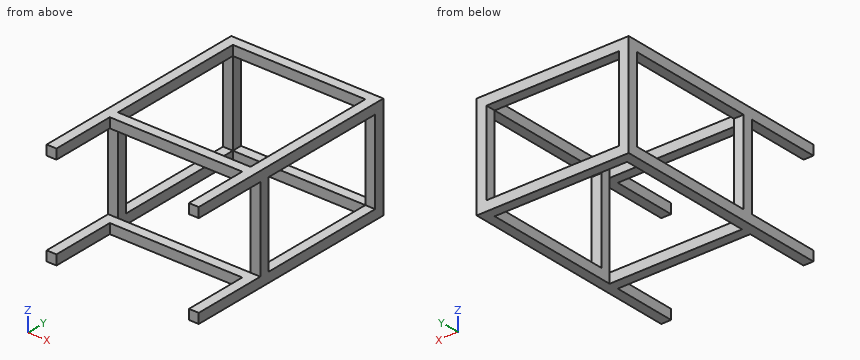
```python
from build123d import *

# Parameters (mm, degrees)
SKETCH_1_W          = 310
SKETCH_1_H          = 210
SKETCH_1_W_2        = 270
SKETCH_1_H_2        = 170
EXTRUDE_1_DEPTH     = 450
SKETCH_8_W          = 170
SKETCH_8_H          = 260
CUT_EXTRUDE_3_DEPTH = 310
SKETCH_11_W         = 170
SKETCH_11_H         = 150
CUT_EXTRUDE_4_DEPTH = 310
SKETCH_13_W         = 270
SKETCH_13_H         = 130
CUT_EXTRUDE_5_DEPTH = 521.216301167
SKETCH_14_W         = 270
SKETCH_14_H         = 280
CUT_EXTRUDE_6_DEPTH = 525.332909515


with BuildPart() as part:
    # 草图1 → 凸台-拉伸1 (new body)
    with BuildSketch(Plane(origin=(0, 0, 0), x_dir=(1, 0, 0), z_dir=(0, 1, 0))):
        Rectangle(SKETCH_1_W, SKETCH_1_H)
        Rectangle(SKETCH_1_W_2, SKETCH_1_H_2, mode=Mode.SUBTRACT)
    extrude(amount=EXTRUDE_1_DEPTH)

    # 草图8 → 切除-拉伸3 (cut)
    with BuildSketch(Plane(origin=(155, 0, 0), x_dir=(0, 0, -1), z_dir=(1, 0, 0))):
        with Locations((0, 300)):
            Rectangle(SKETCH_8_W, SKETCH_8_H)
    extrude(amount=-CUT_EXTRUDE_3_DEPTH, mode=Mode.SUBTRACT)

    # 草图11 → 切除-拉伸4 (cut)
    with BuildSketch(Plane(origin=(155, 0, 0), x_dir=(0, 0, -1), z_dir=(1, 0, 0))):
        with Locations((0, 75)):
            Rectangle(SKETCH_11_W, SKETCH_11_H)
    extrude(amount=-CUT_EXTRUDE_4_DEPTH, mode=Mode.SUBTRACT)

    # 草图13 → 切除-拉伸5 (cut, through all)
    with BuildSketch(Plane.XY.offset(105)):
        with Locations((0, 65)):
            Rectangle(SKETCH_13_W, SKETCH_13_H)
    extrude(amount=-CUT_EXTRUDE_5_DEPTH, mode=Mode.SUBTRACT)

    # 草图14 → 切除-拉伸6 (cut, through all)
    with BuildSketch(Plane.XY.offset(115)):
        with Locations((0, 290)):
            Rectangle(SKETCH_14_W, SKETCH_14_H)
    extrude(amount=-CUT_EXTRUDE_6_DEPTH, mode=Mode.SUBTRACT)


solid = part.part
```
CAD build for the part. Positions are in the model's coordinates, mm. Round coordinates to 2 decimals unless told otherwise and drop trailing zeros. Loops run counter-clockwise (first coordinate to the right, second up) from the corner with the lowest first, then second, coordinate; pieces in that order, holes last. Notation, with made-up numbers: M 28,-39.5 L 33,-39.5 A11 cw 33,-33.5 Z; hole C 72,13.25 d8. An arc over 180 degrees is marked long. Return JSON: item names as keys, results as strings. Group by question number.
(1) Saw through at B-B, the plane y = 274. List the corners of the cut face in (x, z), and give its area (3 significant figures).
(2) Drop a flat-ended pin along its axis: P1, Ø22, axis at x = -145.5, z = -32.5, coming from the -Y side. Give the stop position or say it passes through.
(3) Saw through at A-A, the plane x = -32.5. List the corners of the cut face in (y, z).
(4) Wall check: probe 1 along Z at (x, y) = (139.5, 361); probe 2 along Y at (x, z) = (-139, 38); probe 3 along X at (y, z) = (155, 90). Give the ranges that are in metal, low to high. Write a range as [from, to].
Answer list:
{
 "1": {"outline": "M -155,-105 L -135,-105 L -135,-85 L -155,-85 Z; M -155,85 L -135,85 L -135,105 L -155,105 Z; M 135,-105 L 155,-105 L 155,-85 L 135,-85 Z; M 135,85 L 155,85 L 155,105 L 135,105 Z", "area": "1,600 mm2"},
 "2": {"P1": "y = 150"},
 "3": {"outline": "M 130,-105 L 150,-105 L 150,-85 L 130,-85 Z; M 130,85 L 150,85 L 150,105 L 130,105 Z; M 430,-105 L 450,-105 L 450,-85 L 430,-85 Z; M 430,85 L 450,85 L 450,105 L 430,105 Z"},
 "4": {"probe 1": "[-105, -85], [85, 105]", "probe 2": "[150, 170], [430, 450]", "probe 3": "[-155, -135], [135, 155]"}
}
